Model file for the job. Use its own axes, mm. A direction names the side the tool comes from. Coordinates: 2 decimals unless noted, no trailing zeros. Loops run counter-clockwise (first coordinate to the right, second up) from the corner with the lowest first, then second, coordinate; pieces in that order, holes last. Notation, with made-up numbers: (-7.5, 55.5) -> (48.5, 55.5) arc R28 cw to (48.5, 81.5) -> close; hole circle Ø9 at (-8.75, 75.25). An arc over 180 degrees is marked (long way). Use one line per item in the form item = value.
```python
from build123d import *

# Parameters (mm, degrees)
SKETCH1_R           = 5
BOSS_EXTRUDE1_DEPTH = 85
SKETCH2_R           = 2
CUT_EXTRUDE1_DEPTH  = 15
CUT_EXTRUDE5_DEPTH  = 10
SKETCH6_R           = 2
CUT_EXTRUDE6_DEPTH  = 6


with BuildPart() as part:
    # Sketch1 → Boss-Extrude1 (new body)
    with BuildSketch(Plane(origin=(0, 0, 0), x_dir=(1, 0, 0), z_dir=(0, 1, 0))):
        Circle(SKETCH1_R)
    extrude(amount=BOSS_EXTRUDE1_DEPTH)

    # Sketch2 → Cut-Extrude1 (cut)
    with BuildSketch(Plane(origin=(0, 85, 0), x_dir=(1, 0, 0), z_dir=(0, 1, 0))):
        Circle(SKETCH2_R)
    extrude(amount=-CUT_EXTRUDE1_DEPTH, mode=Mode.SUBTRACT)

    # Sketch3 → Cut-Extrude5 (cut)
    with BuildSketch(Plane.XZ):
        with BuildLine():
            Line((5, 0), (-5, 0))
            ThreePointArc((-5, 0), (0, -5), (5, 0))
        make_face()
    extrude(amount=-CUT_EXTRUDE5_DEPTH, mode=Mode.SUBTRACT)

    # Sketch6 → Cut-Extrude6 (cut, through all)
    with BuildSketch(Plane(origin=(0, 0, 0), x_dir=(-1, 0, 0), z_dir=(0, 0, -1))):
        with Locations((0, 5)):
            Circle(SKETCH6_R)
    extrude(amount=-CUT_EXTRUDE6_DEPTH, mode=Mode.SUBTRACT)


solid = part.part
```
Q1. Pin check, flat tips, straight feed: pin 1 Ø4 at (x, y) = (-3.5, 74) entering from +Z; pin 2 Ø1.5 at (x, z) = (0, -2) entering from -Y; pin 3 Ø1.5 at (y, z) = (64, -3.5) entering from -X. Stop position of each tip, or through.
Result:
pin_1 = 4.77
pin_2 = 10
pin_3 = -4.18
Q2. Wall check: line 1 along Z through (x, y) = (0, 76.75); line 2 along Y through (x, z) = (0, 3.15); line 3 along Y through (x, z) = (-0.5, -0.5). Give the ranges that are in metal, low to high.
Result:
line_1 = -5 to -2, 2 to 5
line_2 = 0 to 3, 7 to 85
line_3 = 10 to 70
Q3. Band-saw the part on C-C, the plane y = 5. Write the cut outline in (x, z).
Result:
outline = (-5, 0) -> (-2, 0) -> (-2, 4.58) arc R5 ccw to start; (2, 0) -> (5, 0) arc R5 ccw to (2, 4.58) -> close
Q4. Band-saw the part on D-D, the plane x = -3.75. Write the cut outline in (y, z).
Result:
outline = (0, 0) -> (10, 0) -> (10, -3.31) -> (85, -3.31) -> (85, 3.31) -> (0, 3.31) -> close
Q5. Band-saw the part on A-A, the plane x = 0. Write the cut outline in (y, z).
Result:
outline = (0, 0) -> (3, 0) -> (3, 5) -> (0, 5) -> close; (7, 0) -> (10, 0) -> (10, -5) -> (85, -5) -> (85, -2) -> (70, -2) -> (70, 2) -> (85, 2) -> (85, 5) -> (7, 5) -> close
Q6. Band-saw the part on B-B, the plane z = 1.25. Write the cut outline in (x, y), and give its area (3 significant figures).
Result:
outline = (-4.84, 0) -> (4.84, 0) -> (4.84, 85) -> (1.56, 85) -> (1.56, 70) -> (-1.56, 70) -> (-1.56, 85) -> (-4.84, 85) -> close; hole circle Ø4 at (0, 5)
area = 764 mm2
Q7. Which spindle directions (+Z, -Z, +X, -X, +Y, -Y) get a long thin tool onto all of the face, cutting with end or side? Do faces 4 (the face through (0, 70, 0)), 5 (the face through (-0.1, 85, 2.2)), 6 (the face through (0, 10, -2)). Say none if no direction does.
Result:
face_4 = +Y
face_5 = +Z, -Z, +X, -X, +Y
face_6 = -Z, +X, -X, -Y
Q8. Mould opens along Z. For faces 1 (the face through (2.307, 41.905, 4.436)), 2 (the face through (0, 78, 2)), 3 (the face through (2, 5, 2)) say: released by +Z, released by -Z, zero draft, split by the parting line, or undercut.
Result:
face_1 = split by the parting line
face_2 = undercut
face_3 = zero draft
